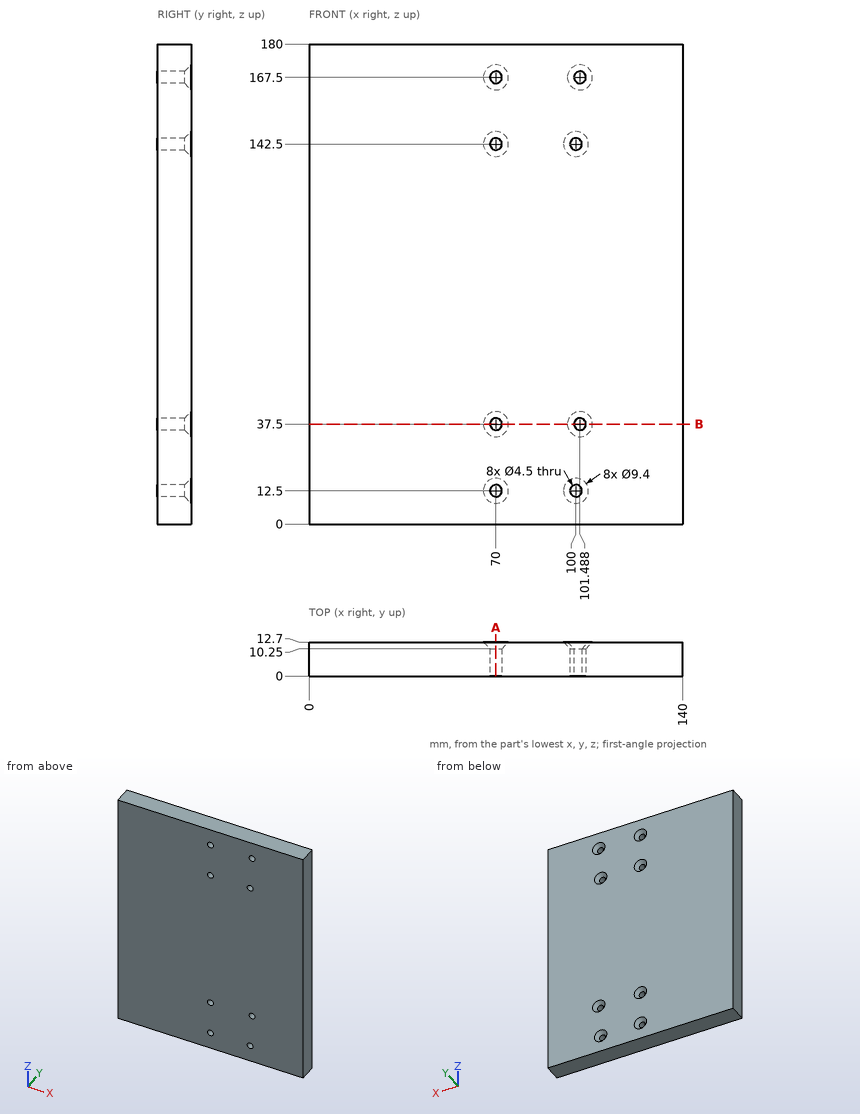
The drawing under review shows one solid part. Ordinate dimensions are in mm from its lowest x, y, z. Give positions to 0.01 mm unless a question says otherwise; leave off trailing zeros. Loops run counter-clockwise (first coordinate to the right, second up) from the corner with the lowest first, then second, coordinate; pieces in that order, holes last. Notation, with made-up numbers: M 44.25,45 L 74.25,45 A34 ccw 74.25,80 Z; hole C -18.5,59.25 d4. An arc over 180 degrees is marked long. One line per item, written item: value. Start each with the question number.
Q1. For L1, parallel to X at y = 4.75, z = 12.5; L2, parallel to Z at x = 70, y = 4.25; L3, parallel to X at y = 5.5, z = 167.5, list the stretches that pass through material, from the lowest coordinate up.
Q2. Add section B-B (z = 37.5). Give the boundary of the cut face in (x, y), and give its area (3 significant figures).
Q3. Clearance check with flat-ended pins moving along their axes: pin 1 Ø4 at (x, z) = (70, 167.5) entering from -Y; pin 2 Ø6 at (x, z) = (70, 142.5) entering from -Y; pin 3 Ø5 at (x, z) = (100, 142.5) entering from +Y; pin 4 Ø6 at (x, z) = (70, 37.5) entering from +Y. State where each tip first meets the part, or that it passes through.
Q4. Add section A-A (x = 70). Give the boundary of the cut face in (y, z).
Reply:
1. L1: 0 to 67.75, 72.25 to 97.75, 102.25 to 140
1. L2: 0 to 10.25, 14.75 to 35.25, 39.75 to 140.25, 144.75 to 165.25, 169.75 to 180
1. L3: 0 to 67.75, 72.25 to 99.24, 103.74 to 140
2. outline: M 0,0 L 67.75,0 L 67.75,10.25 L 65.3,12.7 L 0,12.7 Z; M 72.25,0 L 99.24,0 L 99.24,10.25 L 96.79,12.7 L 74.7,12.7 L 72.25,10.25 Z; M 103.74,0 L 140,0 L 140,12.7 L 106.19,12.7 L 103.74,10.25 Z
2. area: 1,650 mm²
3. pin 1: through
3. pin 2: y = 0
3. pin 3: y = 10.5
3. pin 4: y = 11
4. outline: M 0,0 L 12.7,0 L 12.7,7.8 L 10.25,10.25 L 0,10.25 Z; M 0,14.75 L 10.25,14.75 L 12.7,17.2 L 12.7,32.8 L 10.25,35.25 L 0,35.25 Z; M 0,39.75 L 10.25,39.75 L 12.7,42.2 L 12.7,137.8 L 10.25,140.25 L 0,140.25 Z; M 0,144.75 L 10.25,144.75 L 12.7,147.2 L 12.7,162.8 L 10.25,165.25 L 0,165.25 Z; M 0,169.75 L 10.25,169.75 L 12.7,172.2 L 12.7,180 L 0,180 Z
